```python
from build123d import *
from build123d.topology import SkipClean

# Parameters (mm, degrees)
CHAMFER_1_SIZE          = 1
CUT_EXTRUDE_1_DEPTH     = 76.279479276
EXTRUDE_2_DEPTH         = 16.7
HOLE_WIZARD_M10_1_D     = 8.5
HOLE_WIZARD_M10_1_DEPTH = 27.5
HOLE_WIZARD_M10_1_TIP   = 2.553657631
CHAMFER_2_SIZE          = 0.5


with BuildPart() as part:
    # 草图1 → 旋转1 (revolve)
    with BuildSketch(Plane.XY, mode=Mode.PRIVATE) as revolve_1_sk:
        Polygon((0, 0), (10, 0), (10, 1.9), (9.5, 1.9), (9.5, 3), (10, 3), (10, 63), (13, 63), (13, 73), (9, 73), (9, 93), (0, 93), align=None)
    revolve(revolve_1_sk.sketch.rotate(Axis((0, 0, 0), (0, 1, 0)), 90), axis=Axis((0, 0, 0), (0, 1, 0)))

    # 倒角1
    chamfer_1_edges = [part.edges().sort_by_distance(p)[0] for p in [
        (0, 93, 9),
    ]]
    chamfer(chamfer_1_edges, length=CHAMFER_1_SIZE)

    # 草图2 → 切除-拉伸1 (cut, through all)
    with BuildSketch(Plane(origin=(0, 73, 0), x_dir=(1, 0, 0), z_dir=(0, 1, 0))):
        with BuildLine():
            Line((-11, -6.92820323), (-11, 6.92820323))
            ThreePointArc((-11, 6.92820323), (-13, 0), (-11, -6.92820323))
        make_face()
        with BuildLine():
            ThreePointArc((13, 0), (12.489995997, 3.605551275), (11, 6.92820323))
            Line((11, 6.92820323), (11, -6.92820323))
            ThreePointArc((11, -6.92820323), (12.489995997, -3.605551275), (13, 0))
        make_face()
    extrude(amount=-CUT_EXTRUDE_1_DEPTH, mode=Mode.SUBTRACT)

    # 草图6 → 凸台-拉伸2 (add)
    with SkipClean():  # the faces are left unmerged after this step: merging them gives an invalid solid
        with BuildSketch(Plane.XZ.offset(-63)):
            with BuildLine():
                Line((11, -6.92820323), (11, 6.92820323))
                ThreePointArc((11, 6.92820323), (0, 13), (-11, 6.92820323))
                Line((-11, 6.92820323), (-11, -6.92820323))
                ThreePointArc((-11, -6.92820323), (0, -13), (11, -6.92820323))
            make_face()
        extrude(amount=EXTRUDE_2_DEPTH)

    # M10 螺纹孔1
    with Locations(Plane(origin=(0, 0, 0), x_dir=(-1, 0, 0), z_dir=(0, -1, 0))):
        with Locations((0, 0)):
            Hole(HOLE_WIZARD_M10_1_D / 2, depth=HOLE_WIZARD_M10_1_DEPTH)
            with Locations((0, 0, -(HOLE_WIZARD_M10_1_DEPTH + HOLE_WIZARD_M10_1_TIP / 2))):  # 118° drill point
                Cone(0, HOLE_WIZARD_M10_1_D / 2, HOLE_WIZARD_M10_1_TIP, mode=Mode.SUBTRACT)

    # 倒角2
    chamfer_2_edges = [part.edges().sort_by_distance(p)[0] for p in [
        (0, 0, 10),
    ]]
    chamfer(chamfer_2_edges, length=CHAMFER_2_SIZE)


solid = part.part
```
Input: part model. Units: mm. Frame: model coordinates. A direction names the side the tool comes from. Give positions to 0.01 mm unless a question says otherwise; leave off trailing zeros. Order: outer loops, then holes, each group sorted by start corner. A loop starts at its lowest first (then second) coordinate and runs counter-clockwise, first axis right, second up.
1. Section A-A on y = 34. Return the cut outline in (x, z), and give its area (3 significant figures).
Derived:
outline: circle Ø20 at (0, 0)
area: 314 mm2
2. Pin query (flat end, axial travel): pin 1 (1 mm diameter, centred on x = -7.5, y = 80.5, fed in from +Z); pin 2 (6 mm diameter, centred on x = 0.5, z = 4, fed in from -Y); pin 3 (5 mm diameter, centred on y = 41.5, z = 6.5, fed in from -X); pin 4 (6 mm diameter, centred on x = -2, y = 42.5, fed in from +Z). Return the tip coordinate at first contact, or that it passes through.
Derived:
pin 1: stops at z = 5.66
pin 2: stops at y = 0
pin 3: stops at x = -9.17
pin 4: stops at z = 10
3. Section B-B on y = 68. Return the cut outline in (x, z).
Derived:
outline: (-11, -6.93) arc R13 ccw to (11, -6.93) - (11, 6.93) arc R13 ccw to (-11, 6.93) - close
4. Material intervals for L1, parallel to Y at x = 4.25, z = 9.25; L2, parallel to Z at x = 1.75, y = 23; L3, parallel to Y at x = 9.25, z = 3.25, sorted ascending.
Derived:
L1: y = 46.3 to 73
L2: z = -9.85 to -3.87, 3.87 to 9.85
L3: y = 0.3 to 1.9, 3 to 73
5. Mould query, pull axis Y, two halves, no side actions, for faces 1 (the flat face through (2, 73, 9)), 2 (the cylindrical face through (9.274, 2.458, 2.059)), 3 (the flat face through (4, 3, 9)), 4 (the cylindrical face through (-6.083, 82.633, 6.633)). Classes: released by +Y, released by -Y, zero draft, split by the parting line, or undercut.
Derived:
face 1: released by +Y
face 2: undercut
face 3: undercut
face 4: zero draft
6. Reachability of faces 5 (the flat face through (0, 93, 0)), 6 (the flat face through (4, 1.9, -9)), 7 (the cylindrical face through (0, 25, 10)) from +Z, -Z, +X, -X, +Y, -Y: full face, straight path, thin tool, end or side. Return the list, or none.
Derived:
face 5: +Z, -Z, +X, -X, +Y
face 6: none
face 7: -Y
